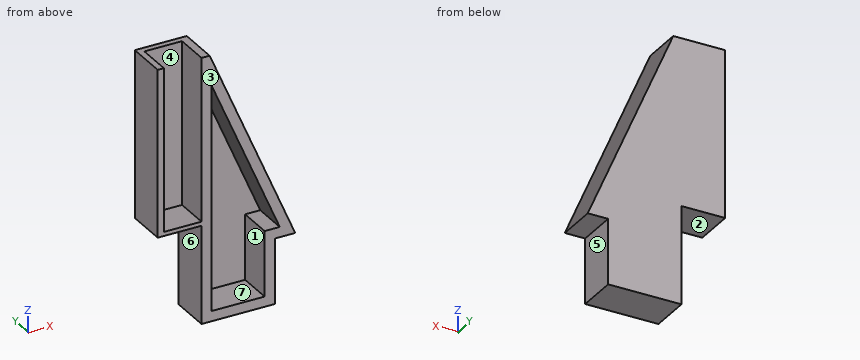
from build123d import *

# Parameters (mm, degrees)
BOSS_EXTRU_1_DEPTH      = 20
BOSS_EXTRU_2_DEPTH      = 85
ESQUISSE4_W             = 50
ESQUISSE4_H             = 20
ENL_V_MAT_EXTRU_1_DEPTH = 47
ENL_V_MAT_EXTRU_2_DEPTH = 17
ESQUISSE6_W             = 21.5
ESQUISSE6_H             = 20
BOSS_EXTRU_3_DEPTH      = 2


with BuildPart() as part:
    # Esquisse1 → Boss.-Extru.1 (new body)
    with BuildSketch(Plane(origin=(0, 0, 0), x_dir=(1, 0, 0), z_dir=(0, 1, 0))):
        Polygon((0, 0), (0, 130), (36, 130), (36, 98), (46, 98), (4, 0), align=None)
    extrude(amount=BOSS_EXTRU_1_DEPTH)

    # Esquisse3 → Boss.-Extru.2 (add)
    with BuildSketch(Plane.XY):
        Polygon((0, 20), (-21.5, 20), (-21.5, 0), (-18.5, 0), (-18.5, 17), (0, 17), align=None)
    extrude(amount=-BOSS_EXTRU_2_DEPTH)

    # Esquisse4 → Enlèv. mat.-Extru.1 (cut)
    with BuildSketch(Plane.ZY):
        with Locations((-105, 10)):
            Rectangle(ESQUISSE4_W, ESQUISSE4_H)
    extrude(amount=ENL_V_MAT_EXTRU_1_DEPTH, mode=Mode.SUBTRACT)

    # Esquisse5 → Enlèv. mat.-Extru.2 (cut)
    with BuildSketch(Plane.XZ):
        Polygon((5, -15.02628851), (5, -125), (31, -125), (31, -93), (38.417304924, -93), align=None)
    extrude(amount=-ENL_V_MAT_EXTRU_2_DEPTH, mode=Mode.SUBTRACT)

    # Esquisse6 → Boss.-Extru.3 (add)
    with BuildSketch(Plane(origin=(0, 0, -80), x_dir=(-1, 0, 0), z_dir=(0, 0, -1))):
        with Locations((10.75, 10)):
            Rectangle(ESQUISSE6_W, ESQUISSE6_H)
    extrude(amount=BOSS_EXTRU_3_DEPTH)


solid = part.part
Geometry check sheet. Reference: the model listing, model coordinates, mm. Face numbers are marked on the shaded views. A direction names the side the tool comes from. Give positions to 0.01 mm unless a question says otherwise; leave off trailing zeros. Loops run counter-clockwise (first coordinate to the right, second up) from the corner with the lowest first, then second, coordinate; pieces in that order, holes last.
(1) Section check C-C on z = -76. Record the cut outline in (x, y).
From the geometry:
outline: (-21.5, 0) - (-18.5, 0) - (-18.5, 17) - (0, 17) - (0, 0) - (5, 0) - (5, 17) - (31.13, 17) - (31.13, 0) - (36.57, 0) - (36.57, 20) - (-21.5, 20) - close
(2) Section check D-D on x = 24. Record the cut outline in (y, z).
From the geometry:
outline: (0, -130) - (20, -130) - (20, -46.67) - (0, -46.67) - (0, -59.36) - (17, -59.36) - (17, -125) - (0, -125) - close
(3) Depth check by flat-ended pin: pin 1 Ø4 at (x, y) = (32.5, 13) entering from +Z; pin 2 Ø5 at (x, y) = (16.5, 9) entering from +Z; pin 3 Ø4 at (x, z) = (-1.5, -62.5) entering from -Y; pin 4 Ø6 at (x, y) = (36.5, 11) entering from +Z. Enter the tip coordinate at first touch or a pass-through.
From the geometry:
pin 1: stops at z = -61.83
pin 2: stops at z = -23.33
pin 3: stops at y = 0
pin 4: stops at z = -68.83
(4) Section check B-B on x = -13. Record the cut outline in (y, z), then the cut area to 3 significant figures.
From the geometry:
outline: (0, -82) - (20, -82) - (20, 0) - (17, 0) - (17, -80) - (0, -80) - close
area: 280 mm2
(5) Set-up check for the marked faces 4, 5, 6 and 7: record each of +Z, -Z, +X, -X, +Y, -Y from which the full face is reachable in a straight line by a thin tool's end or side.
From the geometry:
face 4: +Z, -Y
face 5: -Z, +X, +Y, -Y
face 6: -Z, -X, +Y, -Y
face 7: -Y
(6) Release check for a two-part mould opening along Z. For the marked faces 1, 2 and 3 record: released by +Z, released by -Z, zero draft, split by the parting line, or undercut.
From the geometry:
face 1: undercut
face 2: released by -Z
face 3: zero draft
(7) Section check A-A on y = 8. Record the cut outline in (x, z).
From the geometry:
outline: (-21.5, -82) - (0, -82) - (0, -130) - (36, -130) - (36, -98) - (46, -98) - (4, 0) - (0, 0) - (0, -80) - (-18.5, -80) - (-18.5, 0) - (-21.5, 0) - close; hole (5, -125) - (31, -125) - (31, -93) - (38.42, -93) - (5, -15.03) - close
(8) Thickness scan on L1, parallel to X at y = 3.25, z = -66.5; L2, parallel to X at y = 10.5, z = -25; L3, parallel to X at y = 14, z = -104.5. Record the ranges inside material, lowest first.
From the geometry:
L1: x = -21.5 to -18.5, 0 to 5, 27.06 to 32.5
L2: x = -21.5 to -18.5, 0 to 5, 9.27 to 14.71
L3: x = 0 to 5, 31 to 36
